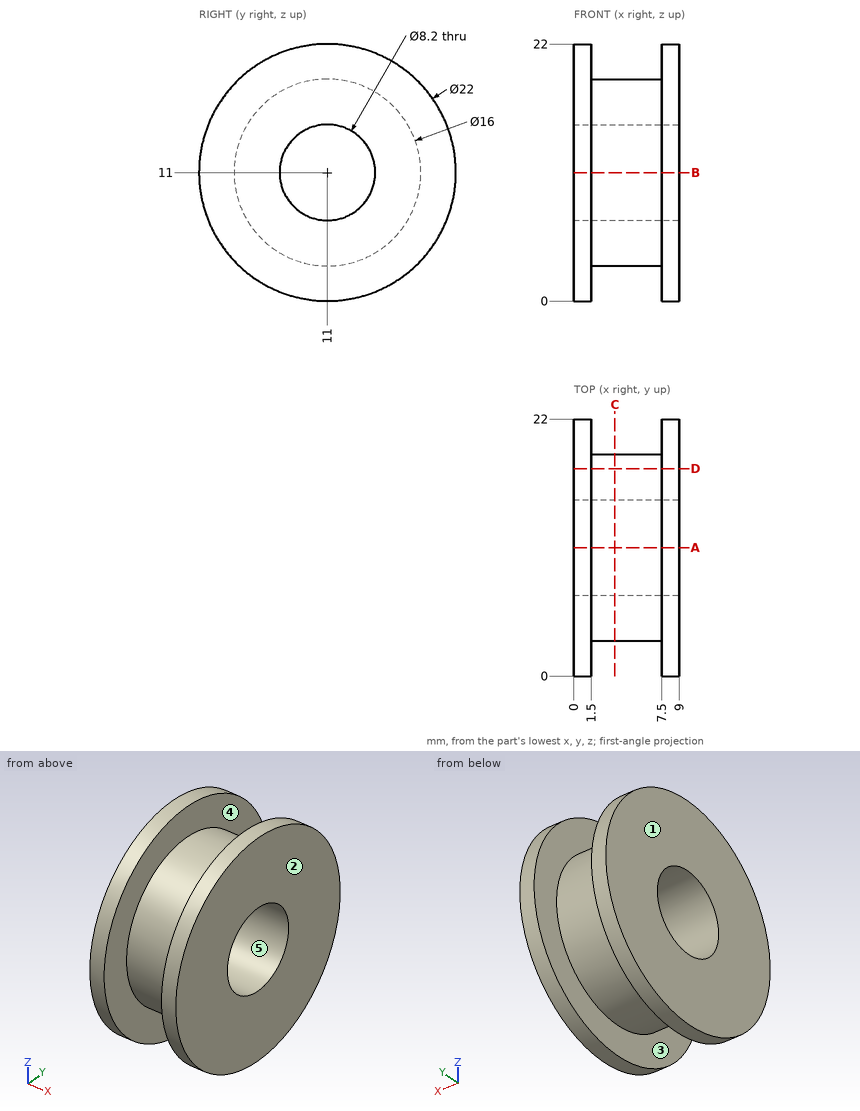
Can you work these out from the drawing? Everything is in mm from the part's minimum corner. A direction names the side the tool comes from. Round coordinates to 2 decimals unless told otherwise and drop trailing zeros. Loops run counter-clockwise (first coordinate to the right, second up) from the corner with the lowest first, then second, coordinate; pieces in that order, holes last. Notation, with made-up numbers: (81, 79.25) -> (139, 79.25) arc R16 cw to (139, 97.25) -> close; hole circle Ø10 at (4.25, 15.25). An arc over 180 degrees is marked (long way). One line per question, with ' | ' between items.
(1) If we section it at C-C on x = 3.5: List the corners of the cut face in (y, z) for me, and give its area (3 significant figures).
Model answer:
outline: circle Ø16 at (11, 11); hole circle Ø8.2 at (11, 11) | area: 148 mm^2
(2) If we section it at D-D on y = 17.75: List the corners of the cut face in (x, z) for me, and give its area (3 significant figures).
Model answer:
outline: (0, 2.31) -> (1.5, 2.31) -> (1.5, 6.71) -> (7.5, 6.71) -> (7.5, 2.31) -> (9, 2.31) -> (9, 19.69) -> (7.5, 19.69) -> (7.5, 15.29) -> (1.5, 15.29) -> (1.5, 19.69) -> (0, 19.69) -> close | area: 104 mm^2
(3) Thinking about a two-plate mould opening in X: for the marked faces 1, 2 and 3, which applies, released by +X, released by -X, zero draft, split by the parting line, or undercut?
Model answer:
face 1: released by -X | face 2: released by +X | face 3: undercut
(4) For the marked faces 4 and 5, which set-ups out of +Z, -Z, +X, -X, +Y, -Y let a thin tool reach every point of the face, with its end or its side?
Model answer:
face 4: none | face 5: +X, -X
(5) If we section it at A-A on y = 11: List the corners of the cut face in (x, z) for me.
Model answer:
outline: (0, 0) -> (1.5, 0) -> (1.5, 3) -> (7.5, 3) -> (7.5, 0) -> (9, 0) -> (9, 6.9) -> (0, 6.9) -> close; (0, 15.1) -> (9, 15.1) -> (9, 22) -> (7.5, 22) -> (7.5, 19) -> (1.5, 19) -> (1.5, 22) -> (0, 22) -> close
(6) If I drill on probe 1 along Z at (x, y) = (4.25, 11); probe 2 along X at (y, z) = (12.75, 1.5), over which ranges is the centre line in solid material (lowest first)?
Model answer:
probe 1: z = 3 to 6.9, 15.1 to 19 | probe 2: x = 0 to 1.5, 7.5 to 9
(7) For pin 1 Ø1.5 at (x, y) = (4.5, 9) entering from -Z; pin 2 Ø5 at (x, z) = (1, 14) entering from -Y; pin 3 Ø5 at (y, z) = (6.5, 8.5) entering from -X, each with a flat end and sliding along its axis, tell me the tip position at first contact or that it passes through.
Model answer:
pin 1: stops at z = 3.1 | pin 2: stops at y = 0.01 | pin 3: stops at x = 0
